from build123d import *

# Parameters (mm, degrees)
SKETCH2_W           = 72
SKETCH2_H           = 47
BOSS_EXTRUDE1_DEPTH = 3
FILLET1_R           = 2
SKETCH3_W           = 66.8
SKETCH3_H           = 41.8
SKETCH3_W_2         = 63.8
SKETCH3_H_2         = 38.8
BOSS_EXTRUDE2_DEPTH = 6
CUT_EXTRUDE1_DEPTH  = 6


with BuildPart() as part:
    # Sketch2 → Boss-Extrude1 (new body)
    with BuildSketch(Plane(origin=(0, 0, 0), x_dir=(1, 0, 0), z_dir=(0, 1, 0))):
        with Locations((36, 23.5)):
            Rectangle(SKETCH2_W, SKETCH2_H)
    extrude(amount=BOSS_EXTRUDE1_DEPTH)

    # Fillet1
    fillet1_edges = [part.edges().sort_by_distance(p)[0] for p in [
        (0, 1.5, 0),
        (72, 1.5, 0),
        (72, 1.5, -47),
        (0, 1.5, -47),
    ]]
    fillet(fillet1_edges, radius=FILLET1_R)

    # Sketch3 → Boss-Extrude2 (add)
    with BuildSketch(Plane(origin=(0, 3, 0), x_dir=(1, 0, 0), z_dir=(0, 1, 0))):
        with Locations((36, 23.5)):
            Rectangle(SKETCH3_W, SKETCH3_H)
        with Locations((36, 23.5)):
            Rectangle(SKETCH3_W_2, SKETCH3_H_2, mode=Mode.SUBTRACT)
    extrude(amount=BOSS_EXTRUDE2_DEPTH)

    # Sketch4 → Cut-Extrude1 (cut)
    with BuildSketch(Plane.XZ):
        with BuildLine():
            Line((14, -9.5), (34, -9.5))
            ThreePointArc((34, -9.5), (36, -11.5), (34, -13.5))
            Line((34, -13.5), (14, -13.5))
            ThreePointArc((14, -13.5), (12, -11.5), (14, -9.5))
        make_face()
    extrude(amount=-CUT_EXTRUDE1_DEPTH, mode=Mode.SUBTRACT)


solid = part.part
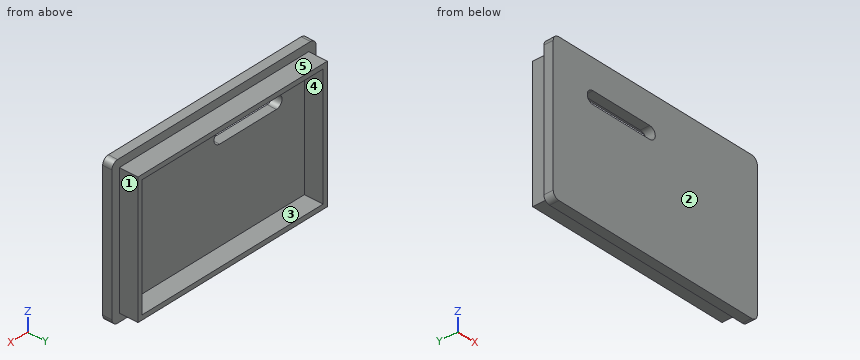
Model file for the job. Use its own axes, mm. Face numbers are marked on the shaded views. A direction names the side the tool comes from. Round coordinates to 2 decimals unless told otherwise and drop trailing zeros. Order: outer loops, then holes, each group sorted by start corner. A loop starts at its lowest first (then second) coordinate and runs counter-clockwise, first axis right, second up.
(1) 3-axis set-ups, long thin cutter, end or side, ignore diameter. For the marked faces 4 and 5: which of +Z, -Z, +X, -X, +Y, -Y reach the whole face in a straight line?
(2) Band-saw the part on C-C (x = 47). List the corners of the cut face in (y, z).
(3) Band-saw the part on D-D (z = -6.5). List the corners of the cut face in (x, y).
(4) Band-saw the part on B-B (z = -11.5). List the corners of the cut face in (x, y).
(5) Pull direction X, two halves, no side cores. Call the marked faces 1, 2 and 3: released by +X, released by -X, zero draft, split by the parting line, or undercut.
(6) Band-saw the part on A-A (y = 7.5). List the corners of the cut face in (x, z), then the cut area to 3 significant figures.
(7) Pin check, flat tips, straight feed: pin 1 (8 mm diameter, centred on x = 50.5, z = -9, fed in from +Y); pin 2 (1 mm diameter, centred on x = 55, y = 5.5, fed in from +Z); pin 3 (3 mm diameter, centred on y = 5.5, z = -24, fed in from +X). Stop position of each tip, or through.
(8) Drill centre lines: line 1 (X direction, y = 8.75, z = -20); line 2 (Z direction, x = 25, y = 7.75); line 3 (Y direction, x = 20.5, z = -6). Where is each one in solid material? Low to high.
Verdict:
1. face 4: +Y
1. face 5: +Z, +X, -X, +Y
2. outline: (0, -47) - (3, -47) - (3, -44.4) - (9, -44.4) - (9, -42.9) - (3, -42.9) - (3, -4.1) - (9, -4.1) - (9, -2.6) - (3, -2.6) - (3, 0) - (0, 0) - close
3. outline: (0, 0) - (72, 0) - (72, 3) - (69.4, 3) - (69.4, 9) - (67.9, 9) - (67.9, 3) - (4.1, 3) - (4.1, 9) - (2.6, 9) - (2.6, 3) - (0, 3) - close
4. outline: (0, 0) - (12, 0) - (12, 3) - (4.1, 3) - (4.1, 9) - (2.6, 9) - (2.6, 3) - (0, 3) - close; (36, 0) - (72, 0) - (72, 3) - (69.4, 3) - (69.4, 9) - (67.9, 9) - (67.9, 3) - (36, 3) - close
5. face 1: released by +X
5. face 2: zero draft
5. face 3: undercut
6. outline: (2.6, -44.4) - (69.4, -44.4) - (69.4, -2.6) - (2.6, -2.6) - close; hole (4.1, -42.9) - (67.9, -42.9) - (67.9, -4.1) - (4.1, -4.1) - close
6. area: 317 mm2
7. pin 1: stops at y = 3
7. pin 2: stops at z = -2.6
7. pin 3: stops at x = 69.4
8. line 1: x = 2.6 to 4.1, 67.9 to 69.4
8. line 2: z = -44.4 to -42.9, -4.1 to -2.6
8. line 3: y = 0 to 3
